Build history of the part. All positions in model axes, mm. Coordinates: 2 decimals unless noted, no trailing zeros. Write each loop counter-clockwise with the first axis right and the second up, starting at its lowest first coordinate (ties: lowest second). Pieces come first, ordered by that corner, then holes.
from build123d import *


with BuildPart() as part:
    # Sketch1 → Revolve1 (revolve)
    with BuildSketch(Plane.XY):
        with BuildLine():
            Line((3, 6), (-3, 6))
            Line((-3, 6), (-6, -6))
            Line((-6, -6), (-3, -6))
            Line((-3, -6), (-1.863803438, -1.45521375))
            ThreePointArc((-1.863803438, -1.45521375), (0, 0), (1.863803438, -1.45521375))
            Line((1.863803438, -1.45521375), (3, -6))
            Line((3, -6), (6, -6))
            Line((6, -6), (3, 6))
        make_face()
    revolve(axis=Axis((-67.31, 0, 0), (0, 1, 0)))


solid = part.part
(1) Slice it at A-A, the plane z = 0. List the corners of the cut face in (x, y), and give its area (3 significant figures).
(2) Two-plate mould, pull along Z, no slides. Class faces 1 (the conical face through (-5.902, -5.716, -19.338)), 2 (the flat face through (-127, -6, 38)), 3 (the conical face through (-128.706, -5.417, -2.702)), 4 (the conical face through (-82.58, 5.42, 68.78)): pulls with the +Z half, pulls with the -Z half, needs draft (parallel to the pull), parting line crosses it, or undercut.
(3) Slice it at B-B, the plane x = -67.31. List the corners of the cut face in (y, z).
(4) Probe L1, parallel to X at y = -5.5, z = 38; L2, parallel to X at y = -3, z = 18.5; L3, parallel to Z at x = -40.5, y = -2. List the from-to ranges inside material, lowest first.
(5) Flat gauge pins, fed straight in: P1, Ø3, axis at y = 4.5, z = 20, coming from the +X side; P2, Ø5, axis at y = 3, z = 16.5, coming from the -X side; P3, Ø6, axis at y = -3.5, z = 50, coming from the -X side. Where does each tip first touch, or does it go through?
(6) Slice it at C-C, the plane y = 2. List the corners of the cut face in (x, z).
Results:
1. outline: (-140.62, -6) - (-137.62, -6) - (-136.48, -1.46) arc R1.92 cw to (-132.76, -1.46) - (-131.62, -6) - (-128.62, -6) - (-131.62, 6) - (-137.62, 6) - close; (-6, -6) - (-3, -6) - (-1.86, -1.46) arc R1.92 cw to (1.86, -1.46) - (3, -6) - (6, -6) - (3, 6) - (-3, 6) - close
1. area: 164 mm2
2. face 1: undercut
2. face 2: needs draft
2. face 3: undercut
2. face 4: parting line crosses it
3. outline: (-6, -73.31) - (6, -70.31) - (6, -64.31) - (-6, -61.31) - (-6, -64.31) - (-1.46, -65.45) arc R1.92 cw to (-1.46, -69.17) - (-6, -70.31) - close; (-6, 61.31) - (6, 64.31) - (6, 70.31) - (-6, 73.31) - (-6, 70.31) - (-1.46, 69.17) arc R1.92 cw to (-1.46, 65.45) - (-6, 64.31) - close
4. L1: x = -129.86 to -126.32, -119.35 to -115.58, -19.04 to -15.27, -8.3 to -4.76
4. L2: x = -137.47 to -134.36, -129.68 to -126.55, -8.07 to -4.94, -0.26 to 2.85
4. L3: z = -67.16 to -63.91, -59.55 to -56.25, 56.25 to 59.55, 63.91 to 67.16
5. P1: stops at x = 1.07
5. P2: stops at x = -137.28
5. P3: stops at x = -122.94
6. outline: circle Ø142.62 at (-67.31, 0); hole circle Ø126.62 at (-67.31, 0)
